Source: CAD feature listing. Evaluate the final solid. Frame: model axes, mm. A direction names the side the tool comes from. Give positions to 0.01 mm unless a question says otherwise; leave off trailing zeros. Order: outer loops, then holes, each group sorted by start corner. A loop starts at its lowest first (then second) coordinate and runs counter-clockwise, first axis right, second up. Notation, with made-up numbers: (66.25, 83) -> (77.25, 83) arc R17 cw to (77.25, 115) -> close; hole circle Ø2 at (11.25, 67). An arc over 180 degrees is marked (long way). Answer in a Markdown table with one row per item.
```python
from build123d import *

# Parameters (mm, degrees)
BOX_W              = 10
BOX_H              = 10
BOX_DEPTH          = 10
SKETCH_W           = 4.4
SKETCH_H           = 4.4
PAD_DEPTH          = 4
PAD_FACE4_W        = 10
PAD_FACE4_H        = 10
POCKET_DEPTH       = 2.5
POCKET_FACE5_W     = 10
POCKET_FACE5_H     = 10
POCKET001_DEPTH    = 2.5
SKETCH001_W        = 5
SKETCH001_H        = 10
PAD001_DEPTH       = 10
SKETCH002_W        = 4.4
SKETCH002_H        = 4.4
PAD002_DEPTH       = 4
PAD002_FACE22_W    = 4.4
PAD002_FACE22_H    = 4.4
POCKET002_DEPTH    = 5
POCKET002_FACE16_W = 5
POCKET002_FACE16_H = 10
POCKET003_DEPTH    = 7.5
POCKET003_FACE15_W = 5
POCKET003_FACE15_H = 10
POCKET004_DEPTH    = 2.5
PAD003_DEPTH       = 5
POCKET005_DEPTH    = 10


with BuildPart() as part:
    # Box → Box (new body)
    with BuildSketch(Plane.XY):
        with Locations((5, 5)):
            Rectangle(BOX_W, BOX_H)
    extrude(amount=BOX_DEPTH)

    # Sketch (on Face6 of BaseFeature) → Pad (new body)
    with BuildSketch(Plane.XY.offset(10)):
        with Locations((5, 5)):
            Rectangle(SKETCH_W, SKETCH_H)
    extrude(amount=PAD_DEPTH)

    # Pad Face4 → Pocket (cut)
    with BuildSketch(Plane(origin=(5, 10, 5), x_dir=(1, 0, 0), z_dir=(0, 1, 0))):
        Rectangle(PAD_FACE4_W, PAD_FACE4_H)
    extrude(amount=-POCKET_DEPTH, mode=Mode.SUBTRACT)

    # Pocket Face5 → Pocket001 (cut)
    with BuildSketch(Plane(origin=(5, 0, 5), x_dir=(-1, 0, 0), z_dir=(0, -1, 0))):
        Rectangle(POCKET_FACE5_W, POCKET_FACE5_H)
    extrude(amount=-POCKET001_DEPTH, mode=Mode.SUBTRACT)

    # Sketch001 (on Face3 of Pocket001) → Pad001 (join)
    with BuildSketch(Plane(origin=(0, 7.5, 0), x_dir=(-1, 0, 0), z_dir=(0, 1, 0))):
        with Locations((-5, 5)):
            Rectangle(SKETCH001_W, SKETCH001_H)
    extrude(amount=PAD001_DEPTH)

    # Sketch002 (on Face6 of Pad001) → Pad002 (join)
    with BuildSketch(Plane.XY.offset(10)):
        with Locations((5, 12.5)):
            Rectangle(SKETCH002_W, SKETCH002_H)
    extrude(amount=PAD002_DEPTH)

    # Pad002 Face22 → Pocket002 (cut)
    with BuildSketch(Plane(origin=(5, 12.5, 14), x_dir=(0, 1, 0), z_dir=(0, 0, 1))):
        Rectangle(PAD002_FACE22_W, PAD002_FACE22_H)
    extrude(amount=-POCKET002_DEPTH, mode=Mode.SUBTRACT)

    # Pocket002 Face16 → Pocket003 (cut)
    with BuildSketch(Plane(origin=(5, 17.5, 5), x_dir=(1, 0, 0), z_dir=(0, 1, 0))):
        Rectangle(POCKET002_FACE16_W, POCKET002_FACE16_H)
    extrude(amount=-POCKET003_DEPTH, mode=Mode.SUBTRACT)

    # Pocket003 Face15 → Pocket004 (cut)
    with BuildSketch(Plane(origin=(5, 10, 5), x_dir=(1, 0, 0), z_dir=(0, 1, 0))):
        Rectangle(POCKET003_FACE15_W, POCKET003_FACE15_H)
    extrude(amount=-POCKET004_DEPTH, mode=Mode.SUBTRACT)

    # Pocket004 Face4 → Pad003 (add)
    with BuildSketch(Plane(origin=(5, 5, 0), x_dir=(0, -1, 0), z_dir=(0, 0, -1))):
        Polygon((2.5, 5), (-2.5, 5), (-2.5, 2.5), (-2.5, -2.5), (-2.5, -5), (2.5, -5), align=None)
    extrude(amount=PAD003_DEPTH)

    # Pad003 Face15 → Pocket005 (cut)
    with BuildSketch(Plane(origin=(5, 5, -5), x_dir=(0, -1, 0), z_dir=(0, 0, -1))):
        Polygon((2.5, 5), (-2.5, 5), (-2.5, 2.5), (-2.5, -2.5), (-2.5, -5), (2.5, -5), align=None)
    extrude(amount=-POCKET005_DEPTH, mode=Mode.SUBTRACT)


solid = part.part
```
(1) Access query for faces 1 (the flat face through (7.2, 5, 12)), 2 (the flat face through (5, 2.8, 12)), 3 (the flat face through (2.8, 5, 12)). Directions: +Z, -Z, +X, -X, +Y, -Y. A direction counts if a zero-diameter tool reaches every point of the face in a straight line with its end or side. Return the directions, or none.
A:
| item | result |
|---|---|
| face 1 | +Z, +X, +Y, -Y |
| face 2 | +Z, +X, -X, -Y |
| face 3 | +Z, -X, +Y, -Y |
(2) Pull-direction query (Z, two-part tool) for faces 4 (the flat face through (5, 5, 5)), 5 (the flat face through (5, 5, 14)), 6 (the flat face through (5, 7.2, 12)); classes: +Z half, -Z half, draft (parallel to the pull), parting line (faces both ways), or undercut.
A:
| item | result |
|---|---|
| face 4 | -Z half |
| face 5 | +Z half |
| face 6 | draft |
(3) Section query B-B (x = 5). Return the cut outline in (y, z), plus the area to 3 significant figures.
A:
| item | result |
|---|---|
| outline | (2.5, 5) -> (7.5, 5) -> (7.5, 10) -> (7.2, 10) -> (7.2, 14) -> (2.8, 14) -> (2.8, 10) -> (2.5, 10) -> close |
| area | 42.6 mm^2 |
(4) Section query D-D (x = 7.75). Return the cut outline in (y, z).
A:
| item | result |
|---|---|
| outline | (2.5, 5) -> (7.5, 5) -> (7.5, 10) -> (2.5, 10) -> close |
(5) First-contact query: pin 1 Ø3 at (y, z) = (6, 13) entering from -X; pin 2 Ø1.2 at (y, z) = (5.5, 11.5) entering from +X; pin 3 Ø2 at (x, z) = (5.5, 12.5) entering from +Y. Flat tips, straight axial feed; report the tip coordinate or a pass-through.
A:
| item | result |
|---|---|
| pin 1 | stops at x = 2.8 |
| pin 2 | stops at x = 7.2 |
| pin 3 | stops at y = 7.2 |
(6) Section query A-A (y = 6.95). Return the cut outline in (x, z), plus the area to 3 significant figures.
A:
| item | result |
|---|---|
| outline | (0, 5) -> (10, 5) -> (10, 10) -> (7.2, 10) -> (7.2, 14) -> (2.8, 14) -> (2.8, 10) -> (0, 10) -> close |
| area | 67.6 mm^2 |
(7) Section query C-C (z = 12.75). Return the cut outline in (x, y).
A:
| item | result |
|---|---|
| outline | (2.8, 2.8) -> (7.2, 2.8) -> (7.2, 7.2) -> (2.8, 7.2) -> close |
(8) Ray query, probe 1 along Z at (x, y) = (9.25, 4.65); probe 2 along X at (y, z) = (3.5, 12.25). Return the intervals inside material, ascending.
A:
| item | result |
|---|---|
| probe 1 | z = 5 to 10 |
| probe 2 | x = 2.8 to 7.2 |
